from build123d import *

# Parameters (mm, degrees)
PAD_DEPTH       = 1.6
SKETCH_W        = 101
SKETCH_H        = 59
SKETCH_W_2      = 1
SKETCH_H_2      = 30
SKETCH_H_3      = 40
PAD001_DEPTH    = 16.6
SKETCH002_W     = 16
SKETCH002_H     = 30
POCKET_DEPTH    = 6
SKETCH003_W     = 16
SKETCH003_H     = 8
POCKET001_DEPTH = 16
SKETCH005_R     = 3.55
SKETCH005_R_2   = 1.95
PAD002_DEPTH    = 6.1
PAD005_DEPTH    = 29.5
POCKET003_DEPTH = 0.6
SKETCH004_R     = 1.95
POCKET002_DEPTH = 6.5


with BuildPart() as part:
    # Sketch001 → Pad (new body)
    with BuildSketch(Plane.XY):
        with BuildLine():
            Line((-51.5, 40.5), (51.5, 40.5))
            ThreePointArc((54.5, 37.5), (53.62132, 39.62132), (51.5, 40.5))
            Line((54.5, 37.5), (54.5, 15))
            ThreePointArc((54.5, 15), (55.37868, 12.87868), (57.5, 12))
            Line((57.5, 12), (69, 12))
            ThreePointArc((70.5, 10.5), (70.06066, 11.56066), (69, 12))
            Line((70.5, 10.5), (70.5, -10.5))
            ThreePointArc((69, -12), (70.06066, -11.56066), (70.5, -10.5))
            Line((69, -12), (57.5, -12))
            ThreePointArc((57.5, -12), (55.37868, -12.87868), (54.5, -15))
            Line((54.5, -15), (54.5, -37.5))
            ThreePointArc((51.5, -40.5), (53.62132, -39.62132), (54.5, -37.5))
            Line((51.5, -40.5), (-51.5, -40.5))
            ThreePointArc((-54.5, -37.5), (-53.62132, -39.62132), (-51.5, -40.5))
            Line((-54.5, -37.5), (-54.5, 37.5))
            ThreePointArc((-51.5, 40.5), (-53.62132, 39.62132), (-54.5, 37.5))
        make_face()
        with BuildLine():
            ThreePointArc((-20, 5), (-25, 0), (-20, -5))
            Line((-20, -5), (20, -5))
            ThreePointArc((20, -5), (25, 0), (20, 5))
            Line((20, 5), (-20, 5))
        make_face(mode=Mode.SUBTRACT)
    extrude(amount=PAD_DEPTH)

    # Sketch → Pad001 (join)
    with BuildSketch(Plane.XY):
        with BuildLine():
            Line((-51.5, 40.5), (51.5, 40.5))
            ThreePointArc((54.5, 37.5), (53.62132, 39.62132), (51.5, 40.5))
            Line((54.5, 37.5), (54.5, 15))
            ThreePointArc((54.5, 15), (55.37868, 12.87868), (57.5, 12))
            Line((57.5, 12), (69, 12))
            ThreePointArc((70.5, 10.5), (70.06066, 11.56066), (69, 12))
            Line((70.5, 10.5), (70.5, -10.5))
            ThreePointArc((69, -12), (70.06066, -11.56066), (70.5, -10.5))
            Line((69, -12), (57.5, -12))
            ThreePointArc((57.5, -12), (55.37868, -12.87868), (54.5, -15))
            Line((54.5, -15), (54.5, -37.5))
            ThreePointArc((51.5, -40.5), (53.62132, -39.62132), (54.5, -37.5))
            Line((51.5, -40.5), (-51.5, -40.5))
            ThreePointArc((-54.5, -37.5), (-53.62132, -39.62132), (-51.5, -40.5))
            Line((-54.5, -37.5), (-54.5, 37.5))
            ThreePointArc((-51.5, 40.5), (-53.62132, 39.62132), (-54.5, 37.5))
        make_face()
        Rectangle(SKETCH_W, SKETCH_H, mode=Mode.SUBTRACT)
        with Locations((-47.5, -9.5)):
            Rectangle(SKETCH_W_2, SKETCH_H_2)
        with Locations((-11.5, -4.5)):
            Rectangle(SKETCH_W_2, SKETCH_H_3)
    extrude(amount=PAD001_DEPTH)

    # Sketch002 (on DatumPlane) → Pocket (cut)
    with BuildSketch(Plane.XY.offset(16.6)):
        with Locations((62.5, 0)):
            Rectangle(SKETCH002_W, SKETCH002_H)
    extrude(amount=-POCKET_DEPTH, mode=Mode.SUBTRACT)

    # Sketch003 (on DatumPlane) → Pocket001 (cut)
    with BuildSketch(Plane.YZ.offset(50.5)):
        with Locations((0, 5.6)):
            Rectangle(SKETCH003_W, SKETCH003_H)
    extrude(amount=POCKET001_DEPTH, mode=Mode.SUBTRACT)

    # Sketch005 → Pad002 (join)
    with BuildSketch(Plane.XY):
        with Locations((13.5, -21.5)):
            Circle(SKETCH005_R)
        with Locations((13.5, -21.5)):
            Circle(SKETCH005_R_2, mode=Mode.SUBTRACT)
        with Locations((35.5, -21.5)):
            Circle(SKETCH005_R)
        with Locations((35.5, -21.5)):
            Circle(SKETCH005_R_2, mode=Mode.SUBTRACT)
    extrude(amount=PAD002_DEPTH)

    # Sketch010 → Pad005 (join, symmetric)
    with BuildSketch(Plane.XZ):
        Polygon((44.5, 16.6), (50.5, 16.6), (50.5, 9.6), (44.5, 15.6), align=None)
        Polygon((-50.5, 16.6), (-44.5, 16.6), (-44.5, 15.6), (-50.5, 9.6), align=None)
    extrude(amount=PAD005_DEPTH, both=True)

    # Sketch006 (on DatumPlane) → Pocket003 (cut)
    with BuildSketch(Plane.XY.offset(16.6)):
        with BuildLine():
            Line((-43.5, 32), (43.5, 32))
            ThreePointArc((47, 28.5), (45.974874, 30.974874), (43.5, 32))
            Line((47, 28.5), (47, -28.5))
            ThreePointArc((43.5, -32), (45.974874, -30.974874), (47, -28.5))
            Line((43.5, -32), (-43.5, -32))
            ThreePointArc((-47, -28.5), (-45.974874, -30.974874), (-43.5, -32))
            Line((-47, -28.5), (-47, 28.5))
            ThreePointArc((-43.5, 32), (-45.974874, 30.974874), (-47, 28.5))
        make_face()
        with BuildLine():
            Line((-43.5, 31), (43.5, 31))
            ThreePointArc((46, 28.5), (45.267767, 30.267767), (43.5, 31))
            Line((46, 28.5), (46, -28.5))
            ThreePointArc((43.5, -31), (45.267767, -30.267767), (46, -28.5))
            Line((43.5, -31), (-43.5, -31))
            ThreePointArc((-46, -28.5), (-45.267767, -30.267767), (-43.5, -31))
            Line((-46, -28.5), (-46, 28.5))
            ThreePointArc((-43.5, 31), (-45.267767, 30.267767), (-46, 28.5))
        make_face(mode=Mode.SUBTRACT)
    extrude(amount=-POCKET003_DEPTH, mode=Mode.SUBTRACT)

    # Sketch004 (on DatumPlane) → Pocket002 (cut)
    with BuildSketch(Plane.XY.offset(16.6)):
        with Locations((-50.55, 36.55)):
            Circle(SKETCH004_R)
        with Locations((-10.55, 36.55)):
            Circle(SKETCH004_R)
        with Locations((10.55, 36.55)):
            Circle(SKETCH004_R)
        with Locations((50.55, 36.55)):
            Circle(SKETCH004_R)
        with Locations((50.55, -36.55)):
            Circle(SKETCH004_R)
        with Locations((10.55, -36.55)):
            Circle(SKETCH004_R)
        with Locations((-10.55, -36.55)):
            Circle(SKETCH004_R)
        with Locations((-50.55, -36.55)):
            Circle(SKETCH004_R)
        with Locations((-50.55, 0)):
            Circle(SKETCH004_R)
        with Locations((50.55, 0)):
            Circle(SKETCH004_R)
    extrude(amount=-POCKET002_DEPTH, mode=Mode.SUBTRACT)


solid = part.part
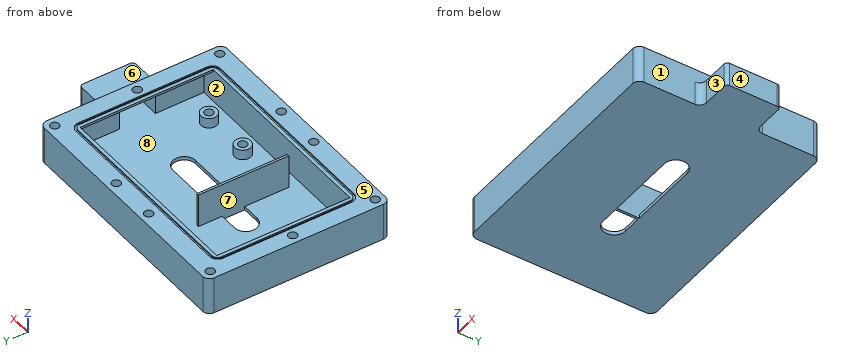
Source: CAD feature listing. Evaluate the final solid. Frame: model axes, mm. Face numbers are marked on the shaded views. A direction names the side the tool comes from. Coordinates: 2 decimals unless noted, no trailing zeros. Write each loop counter-clockwise with the first axis right and the second up, starting at its lowest first coordinate (ties: lowest second). Pieces come first, ordered by that corner, then holes. Notation, with made-up numbers: M 59.5,-35.5 L 98.5,-35.5 A19 ccw 98.5,-16.5 Z; hole C 2.5,8.5 d6. An arc over 180 degrees is marked long. Use a Markdown table: item, result.
1) First-contact query: pin 1 Ø2.5 at (x, z) = (59.5, 5) entering from -Y; pin 2 Ø8 at (x, y) = (36.5, -22.5) entering from +Z. Flat tips, straight axial feed; report the tip coordinate or a pass-through.
Conclusion:
| item | result |
|---|---|
| pin 1 | stops at y = -12 |
| pin 2 | stops at z = 6.1 |
2) Section A-A, the plane x = 60. Output: boundary loops of the cut face in (y, z), then the cut area to 3 significant figures.
Conclusion:
| item | result |
|---|---|
| outline | M -12,0 L 12,0 L 12,10.6 L -12,10.6 Z; hole M -8,1.6 L 8,1.6 L 8,9.6 L -8,9.6 Z |
| area | 126 mm^2 |
3) Ray query, L1, parallel to Y at x = 13.5, z = 4.65; L2, parallel to Y at x = -10.55, z = 12.25; L3, parallel to Y at x = -43, z = 9. Return the intervals inside material, ascending.
Conclusion:
| item | result |
|---|---|
| L1 | y = -40.5 to -29.5, -25.05 to -23.45, -19.55 to -17.95, 29.5 to 40.5 |
| L2 | y = -40.5 to -38.5, -34.6 to -29.5, 29.5 to 34.6, 38.5 to 40.5 |
| L3 | y = -40.5 to -29.5, 29.5 to 40.5 |
4) Mould query, pull axis Y, two halves, no side actions, for the marked faces 1, 2 and 3. Classes: pulls with the +Y half, pulls with the -Y half, needs draft (parallel to the pull), parting line crosses it, or undercut.
Conclusion:
| item | result |
|---|---|
| face 1 | needs draft |
| face 2 | undercut |
| face 3 | pulls with the -Y half |
5) Section B-B, the plane y = 18.5. Output: boundary loops of the cut face in (x, z), then the cut area to 3 significant figures.
Conclusion:
| item | result |
|---|---|
| outline | M -54.5,0 L 54.5,0 L 54.5,16.6 L 47,16.6 L 47,16 L 46,16 L 46,16.6 L 44.5,16.6 L 44.5,15.6 L 50.5,9.6 L 50.5,1.6 L -50.5,1.6 L -50.5,9.6 L -44.5,15.6 L -44.5,16.6 L -46,16.6 L -46,16 L -47,16 L -47,16.6 L -54.5,16.6 Z |
| area | 341 mm^2 |
6) Reachability of the marked faces 4, 5, 6, 7 and 8 from +Z, -Z, +X, -X, +Y, -Y: full face, straight path, thin tool, end or side. Return the list, or none.
Conclusion:
| item | result |
|---|---|
| face 4 | +Z, -Z, +X, +Y, -Y |
| face 5 | +Z, +X, -X, +Y, -Y |
| face 6 | +Z, +X, +Y, -Y |
| face 7 | +Z |
| face 8 | none |
